Could you check a few things on this model? Use its own coordinates, in mm. A direction names the side the tool comes from. Coordinates: 2 decimals unless noted, no trailing zeros. Loops run counter-clockwise (first coordinate to the right, second up) from the corner with the lowest first, then second, coordinate; pieces in that order, holes last. Notation, with made-up numbers: M -23.5,-5 L 31.5,-5 A21 ccw 31.5,11 Z; hole C -21,10.5 d7. An arc over 180 degrees is marked long. Write each question's results on one line, items separated by ' | '.
```python
from build123d import *

# Parameters (mm, degrees)
SKETCH_R      = 28.5
PAD_DEPTH     = 1.6
SKETCH001_R   = 28.5
SKETCH001_R_2 = 27.7
PAD001_DEPTH  = 20
FILLET_R      = 0.5
FILLET001_R   = 1


with BuildPart() as part:
    # Sketch → Pad (new body)
    with BuildSketch(Plane.XY):
        Circle(SKETCH_R)
    extrude(amount=PAD_DEPTH)

    # Sketch001 (on Face3 of Pad) → Pad001 (join)
    with BuildSketch(Plane.XY.offset(1.6)):
        Circle(SKETCH001_R)
        Circle(SKETCH001_R_2, mode=Mode.SUBTRACT)
    extrude(amount=PAD001_DEPTH)

    # Fillet
    fillet_edges = [part.edges().sort_by_distance(p)[0] for p in [
        (-28.5, 0, 0),
    ]]
    fillet(fillet_edges, radius=FILLET_R)

    # Fillet001
    fillet001_edges = [part.edges().sort_by_distance(p)[0] for p in [
        (-27.7, 0, 1.6),
    ]]
    fillet(fillet001_edges, radius=FILLET001_R)


solid = part.part
```
(1) If we mould it in two halves opening along Y, with no side actions, what happens to faces 1 (the cylindrical face through (26.327, -10.916, 10.902)), 2 (the flat face through (-4, 28, 21.6)), 3 (the flat face through (0, 0, 1.6))? For each: released by +Y, released by -Y, zero draft, split by the parting line, or undercut.
Reported:
face 1: split by the parting line | face 2: zero draft | face 3: undercut
(2) Which directions (+Z, -Z, +X, -X, +Y, -Y) give clear straight access to the entire face, cutting with the end or side of a thin tool? Please do faces 4 (the flat face through (0, 0, 0)), 5 (the cylindrical face through (26.42, 8.32, 11.97)).
Reported:
face 4: -Z, +X, -X, +Y, -Y | face 5: +Z
(3) Will these pins go through, and if not, where does the flat tip stop? P1, Ø8, axis at y = 6, z = 19, coming from the -X side; P2, Ø1, axis at x = 22, z = 14.5, coming from the +Y side; P3, Ø6, axis at y = 15, z = 5, coming from the +X side; P4, Ø4, axis at x = 3, y = -13.5, coming from the -Z side.
Reported:
P1: stops at x = -28.43 | P2: stops at y = 18.71 | P3: stops at x = 25.85 | P4: stops at z = 0
(4) Imagine slicing it at A-A, the plane y = 0. List the corners of the cut face in (x, z) for me.
Reported:
outline: M -28.5,0.5 A0.5 ccw -28,0 L 28,0 A0.5 ccw 28.5,0.5 L 28.5,21.6 L 27.7,21.6 L 27.7,2.6 A1 cw 26.7,1.6 L -26.7,1.6 A1 cw -27.7,2.6 L -27.7,21.6 L -28.5,21.6 Z
(5) Imagine slicing it at C-C, the plane z = 11.25. List the corners of the cut face in (x, y) for me, and give its area (3 significant figures).
Reported:
outline: C 0,0 d57; hole C 0,0 d55.4 | area: 141 mm2
(6) Please list where these lines run through material, in increasing order: probe 1 along Y at (x, z) = (0, 15.75); probe 2 along Z at (x, y) = (0, -10); probe 3 along Y at (x, z) = (-10.5, 16.75). Write a range as from..to.
Reported:
probe 1: y = -28.5..-27.7, 27.7..28.5 | probe 2: z = 0..1.6 | probe 3: y = -26.5..-25.63, 25.63..26.5
